Read the model definition and answer for the solid it produces. Units are mm, in the model's axes. Face numbers are marked on the shaded views. A direction names the side the tool comes from. Coordinates: 2 decimals unless noted, no trailing zeros. Write each loop counter-clockwise with the first axis right and the second up, starting at its lowest first coordinate (ties: lowest second). Pieces come first, ordered by that corner, then holes. Notation, with made-up numbers: (87.25, 18.5) -> (115.25, 18.5) arc R18 cw to (115.25, 45.5) -> close; hole circle Ø1 at (-40, 88). An arc over 180 degrees is marked (long way). Use CSV: the item, a comma, the result in double quotes. Start each with the question number.
Autodesk Inventor part; units mm, degrees
ref_plane "YZ Plane" through (0, 0, 0) normal (1, 0, 0) x (0, 1, 0)
ref_plane "XZ Plane" through (0, 0, 0) normal (0, 1, 0) x (-1, 0, 0)
ref_plane "XY Plane" through (0, 0, 0) normal (0, 0, 1) x (1, 0, 0)
sketch "Sketch1" plane through (0, 0, 0) normal (0, 0, 1) x (1, 0, 0)
  line L0 (0, 0) -> (76.2, 0)
  line L1 (76.2, 0) -> (76.2, 127)
  line L2 (76.2, 127) -> (0, 127)
  line L3 (0, 127) -> (0, 0)
  dimension "d0" = 76.2
  dimension "d1" = 127
extrude "Extrusion1" add sketch "Sketch1" along normal blind 12.7
sketch "Sketch2" plane through (0, 0, 12.7) normal (0, 0, 1) x (1, 0, 0)
  line L0 (0, 0) -> (76.4787, 0)
  line L1 (76.4787, 0) -> (76.4787, 38.1)
  line L2 (76.4787, 38.1) -> (0, 38.1)
  line L3 (0, 38.1) -> (0, 0)
  dimension "d4" = 38.1
extrude "Extrusion2" add sketch "Sketch2" along normal blind 12.7
sketch "Sketch3" plane through (0, 0, 12.7) normal (0, 0, 1) x (1, 0, 0)
  circle A0 centre (25.4, 101.6) radius 9.525
  line L0 (0, 127) -> (0, 38.1)
  line L1 (76.2, 127) -> (0, 127)
  point P0 (0, 0)
  dimension "d7" = 19.05
  dimension "d8" = 25.4
  dimension "d9" = 25.4
extrude "Extrusion3" cut sketch "Sketch3" against normal through all
sketch "Sketch4" plane through (0, 127, 0) normal (0, 1, 0) x (1, 0, 0)
  point P0 (0, 0)
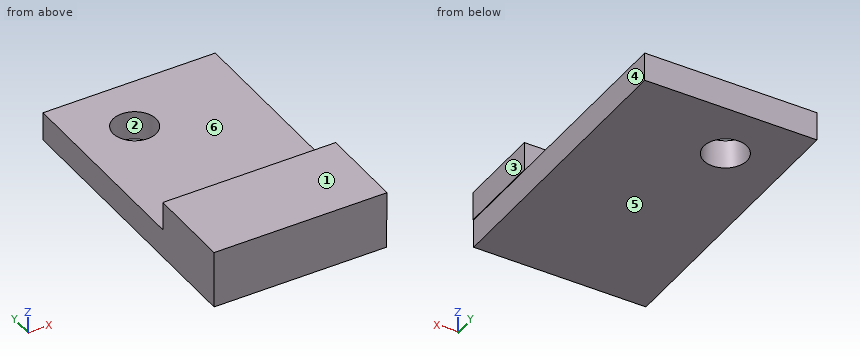
1) Section C-C, the plane z = 5.25 is taken. Give the vertices of the cut face in (x, y) (3 decimals).
2) Section A-A, the plane y = 101.6 is taken. Give the vertices of the cut face in (x, z) (3 decimals).
3) Each of these flat-tipped pins is pushed along its axis until it touches: pin 1 (8 mm diameter, centred on y = 104, z = 5.5, fed in from -X); pin 2 (8 mm diameter, centred on x = 23.5, y = 45.5, fed in from +Z); pin 3 (4 mm diameter, centred on x = 21.5, z = 16.5, fed in from +Y); pin 4 (4 mm diameter, centred on y = 57.5, z = 9, fed in from +X). Where does it stop, or does it pass through?
4) The mould has two halves that part along X. Classify the marked faces 1, 2 and 3: pulls with the +X half, pulls with the -X half, needs draft (parallel to the pull), parting line crosses it, or undercut.
5) Section D-D, the plane x = 48.5 is taken. Give the vertices of the cut face in (y, z).
6) Section B-B, the plane x = 25.4 is taken. Give the vertices of the cut face in (y, z) (3 decimals), plus the area to 3 significant figures.
7) Find the intervals of material crossed by line 1 along Y through (x, z) = (25.4, 8) (3 decimals); line 2 along Y through (x, z) = (55, 24.25); line 3 along X through (y, z) = (72, 2), in increasing order.
8) Which of the six approach directions +Z, -Z, +X, -X, +Y, -Y give full straight-line access (tool end or side, diameter ignored) to the marked faces 4, 5 and 6?
The answers:
1,outline,"(0, 0) -> (76.2, 0) -> (76.2, 127) -> (0, 127) -> close; hole circle Ø19.05 at (25.4, 101.6)"
2,outline,"(0, 0) -> (15.875, 0) -> (15.875, 12.7) -> (0, 12.7) -> close; (34.925, 0) -> (76.2, 0) -> (76.2, 12.7) -> (34.925, 12.7) -> close"
3,pin 1,"stops at x = 0"
3,pin 2,"stops at z = 12.7"
3,pin 3,"stops at y = 38.1"
3,pin 4,"stops at x = 76.2"
4,face 1,"needs draft"
4,face 2,"undercut"
4,face 3,"pulls with the +X half"
5,outline,"(0, 0) -> (127, 0) -> (127, 12.7) -> (38.1, 12.7) -> (38.1, 25.4) -> (0, 25.4) -> close"
6,outline,"(0, 0) -> (92.075, 0) -> (92.075, 12.7) -> (38.1, 12.7) -> (38.1, 25.4) -> (0, 25.4) -> close; (111.125, 0) -> (127, 0) -> (127, 12.7) -> (111.125, 12.7) -> close"
6,area,"1,850 mm^2"
7,line 1,"y = 0 to 92.075, 111.125 to 127"
7,line 2,"y = 0 to 38.1"
7,line 3,"x = 0 to 76.2"
8,face 4,"-Z, +X, +Y, -Y"
8,face 5,"-Z, +X, -X, +Y, -Y"
8,face 6,"+Z, +X, -X, +Y"
